from build123d import *

# Parameters (mm, degrees)
SKETCH2_W               = 35
SKETCH2_H               = 125
SKETCH2_W_2             = 11
SKETCH2_H_2             = 101
BOSS_EXTRUDE1_DEPTH     = 1400
SKETCH3_R               = 6
CUT_EXTRUDE1_DEPTH      = 1407.004978654
SKETCH4_W               = 250
SKETCH4_H               = 150
BOSS_EXTRUDE2_DEPTH     = 12
SKETCH5_W               = 250
SKETCH5_H               = 150
BOSS_EXTRUDE3_DEPTH     = 12
BOSS_EXTRUDE4_START     = -62.5
BOSS_EXTRUDE4_DEPTH     = 6
SKETCH8_R               = 6
CUT_EXTRUDE2_DEPTH      = 12
CUT_EXTRUDE3_DEPTH      = 1426.81783549
CUT_EXTRUDE3_DEPTH_BACK = 1426.81783549


with BuildPart() as part:
    # Sketch2 → Boss-Extrude1 (new body)
    with BuildSketch(Plane(origin=(0, 0, 0), x_dir=(1, 0, 0), z_dir=(0, 1, 0))):
        with Locations((17.5, 62.5)):
            Rectangle(SKETCH2_W, SKETCH2_H)
        with Locations((17.5, 62.5)):
            Rectangle(SKETCH2_W_2, SKETCH2_H_2, mode=Mode.SUBTRACT)
    extrude(amount=BOSS_EXTRUDE1_DEPTH)

    # Sketch3 → Cut-Extrude1 (cut, through all)
    with BuildSketch(Plane(origin=(35, 0, 0), x_dir=(0, 0, -1), z_dir=(1, 0, 0))):
        with Locations((62.5, 950)):
            Circle(SKETCH3_R)
        with Locations((62.5, 900)):
            Circle(SKETCH3_R)
        with Locations((105.801270189, 925)):
            Circle(SKETCH3_R)
        with Locations((37.5, 750)):
            Circle(SKETCH3_R)
        with Locations((87.5, 750)):
            Circle(SKETCH3_R)
        with Locations((105.801270189, 575)):
            Circle(SKETCH3_R)
        with Locations((62.5, 600)):
            Circle(SKETCH3_R)
        with Locations((62.5, 550)):
            Circle(SKETCH3_R)
    extrude(amount=-CUT_EXTRUDE1_DEPTH, mode=Mode.SUBTRACT)

    # Sketch4 → Boss-Extrude2 (add)
    with BuildSketch(Plane(origin=(0, 0, 0), x_dir=(-1, 0, 0), z_dir=(0, -1, 0))):
        with Locations((-17.5, 62.5)):
            Rectangle(SKETCH4_W, SKETCH4_H)
    extrude(amount=BOSS_EXTRUDE2_DEPTH)

    # Sketch5 → Boss-Extrude3 (add)
    with BuildSketch(Plane(origin=(0, 1400, 0), x_dir=(1, 0, 0), z_dir=(0, 1, 0))):
        with Locations((17.5, 62.5)):
            Rectangle(SKETCH5_W, SKETCH5_H)
    extrude(amount=BOSS_EXTRUDE3_DEPTH)

    # Sketch7 → Boss-Extrude4 (add, symmetric)
    with BuildSketch(Plane(origin=(0, 0, -125), x_dir=(-1, 0, 0), z_dir=(0, 0, -1)).offset(BOSS_EXTRUDE4_START)):
        Polygon((-35, 0), (-35, 125), (-142.5, 0), align=None)
        Polygon((0, 125), (107.5, 0), (0, 0), align=None)
    extrude(amount=BOSS_EXTRUDE4_DEPTH, both=True)

    # Sketch8 → Cut-Extrude2 (cut)
    with BuildSketch(Plane(origin=(0, 0, 0), x_dir=(1, 0, 0), z_dir=(0, 1, 0))):
        with Locations(Location((-53.75, 28.25, 0), (0, 0, 270))):
            Circle(SKETCH8_R)
        with Locations(Location((-53.75, 96.75, 0), (0, 0, 270))):
            Circle(SKETCH8_R)
        with Locations(Location((88.75, 28.25, 0), (0, 0, 270))):
            Circle(SKETCH8_R)
        with Locations(Location((88.75, 96.75, 0), (0, 0, 270))):
            Circle(SKETCH8_R)
    extrude(amount=-CUT_EXTRUDE2_DEPTH, mode=Mode.SUBTRACT)

    # Sketch9 → Cut-Extrude3 (cut, two sides: drawn at the far end of the back side and taken through both)
    with BuildSketch(Plane(origin=(35, 0, 0), x_dir=(0, 0, -1), z_dir=(1, 0, 0)).offset(-CUT_EXTRUDE3_DEPTH_BACK)):
        with BuildLine():
            Line((-163.728557717, 1439.709556919), (272.302726902, 1439.709556919))
            Line((272.302726902, 1439.709556919), (272.302726902, 682.852602279))
            Line((272.302726902, 682.852602279), (125, 682.852602279))
            Line((125, 682.852602279), (125, 956))
            ThreePointArc((125, 956), (62.5, 1018.5), (0, 956))
            Line((0, 956), (0, 682.852602279))
            Line((0, 682.852602279), (-163.728557717, 682.852602279))
            Line((-163.728557717, 682.852602279), (-163.728557717, 1439.709556919))
        make_face()
    extrude(amount=CUT_EXTRUDE3_DEPTH + CUT_EXTRUDE3_DEPTH_BACK, mode=Mode.SUBTRACT)


solid = part.part
Here's how the part is built. I have some questions about the finished solid (model axes, mm). A direction names the side the tool comes from. Coordinates: 2 decimals unless noted, no trailing zeros. Write each loop counter-clockwise with the first axis right and the second up, starting at its lowest first coordinate (ties: lowest second). Pieces come first, ordered by that corner, then holes.
1) Which directions (+Z, -Z, +X, -X, +Y, -Y) give clear straight access to the entire face, cutting with the end or side of a thin tool? Please do faces 1 (the face through (17, 471, -125)), 2 (the face through (66, 36, -68.5)), 3 (the face through (23, 502, -62)), 4 (the face through (-31, 36, -68.5)).
Filled in:
face 1: -Z, +X, -X, +Y
face 2: -Z, +X, +Y
face 3: +Y
face 4: -Z, -X, +Y
2) If we section it at D-D (x = 103.5): List the corners of the cut face in (y, z) for me.
Filled in:
outline: (-12, -137.5) - (0, -137.5) - (0, -68.5) - (45.35, -68.5) - (45.35, -56.5) - (0, -56.5) - (0, 12.5) - (-12, 12.5) - close
3) Thinking about a two-plate mould opening in Z: for faces 5 (the face through (-31, 36, -56.5)), 6 (the face through (19, 0, -126)), 7 (the face through (12, 502, -62)), which applies, +Z half, -Z half, draft (parallel to the pull), parting line (faces both ways), or undercut?
Filled in:
face 5: +Z half
face 6: draft
face 7: undercut
4) If we section it at C-C (y = 50.5): List the corners of the cut face in (x, z) for me.
Filled in:
outline: (-64.07, -68.5) - (0, -68.5) - (0, -125) - (35, -125) - (35, -68.5) - (99.07, -68.5) - (99.07, -56.5) - (35, -56.5) - (35, 0) - (0, 0) - (0, -56.5) - (-64.07, -56.5) - close; hole (12, -113) - (23, -113) - (23, -12) - (12, -12) - close
5) If we section it at B-B (x = 53): List the corners of the cut face in (y, z) for me, plus the area to 3 significant figures.
Filled in:
outline: (-12, -137.5) - (0, -137.5) - (0, -68.5) - (104.07, -68.5) - (104.07, -56.5) - (0, -56.5) - (0, 12.5) - (-12, 12.5) - close
area: 3,050 mm2
6) If I drill on line 1 (Y direction, x = 5.25, z = -62.5); line 2 (X direction, y = -7, z = -28); line 3 (X direction, y = 859, z = -29.5), over which ranges is the centre line in solid material (lowest first)?
Filled in:
line 1: y = -12 to 544, 556 to 594, 606 to 894, 906 to 944, 956 to 1018.5
line 2: x = -107.5 to -59.74, -47.76 to 82.76, 94.74 to 142.5
line 3: x = 0 to 12, 23 to 35
7) I'm going to push flat-ended pins straight in: pin 1 (2 mm diameter, centred on y = 337, z = -53, fed in from +X); pin 2 (1.5 mm diameter, centred on y = 130.5, z = -27.5, fed in from -X); pin 3 (3.5 mm diameter, centred on x = 16, z = -39, fed in from +Y). Where does each tip first touch, or does it pass through?
Filled in:
pin 1: stops at x = 35
pin 2: stops at x = 0
pin 3: stops at y = 0
8) If we section it at A-A (y = 337): List the corners of the cut face in (x, z) for me.
Filled in:
outline: (0, -125) - (35, -125) - (35, 0) - (0, 0) - close; hole (12, -113) - (23, -113) - (23, -12) - (12, -12) - close
